from build123d import *

# Parameters (mm, degrees)
EXTRUDE_THIN1_DEPTH = 254
FILLET1_R           = 0.889


with BuildPart() as part:
    # Sketch1 → Extrude-Thin1 (new body)
    with BuildSketch(Plane.XY):
        with BuildLine():
            Line((0, 3.175), (0, 0))
            Line((0, 0), (-4.7625, 0))
            ThreePointArc((-4.7625, 0), (-6.154789008, 7.270660772), (-8.588987157, 14.261773425))
            ThreePointArc((-8.588987157, 14.261773425), (-11.515725494, 17.745797222), (-15.875, 19.05))
            Line((-15.875, 19.05), (-15.875, 25.4))
            Line((-15.875, 25.4), (0, 25.4))
            Line((0, 25.4), (0, 22.225))
            Line((0, 22.225), (-0.889, 22.225))
            Line((-0.889, 22.225), (-0.889, 24.511))
            Line((-0.889, 24.511), (-14.986, 24.511))
            Line((-14.986, 24.511), (-14.986, 19.894116096))
            ThreePointArc((-14.986, 19.894116096), (-10.661715447, 18.234912963), (-7.772953719, 14.614492048))
            ThreePointArc((-7.772953719, 14.614492048), (-5.400232677, 7.883084139), (-3.977402872, 0.889))
            Line((-3.977402872, 0.889), (-0.889, 0.889))
            Line((-0.889, 0.889), (-0.889, 3.175))
            Line((-0.889, 3.175), (0, 3.175))
        make_face()
    extrude(amount=-EXTRUDE_THIN1_DEPTH)

    # Fillet1
    fillet1_edges = [part.edges().sort_by_distance(p)[0] for p in [
        (0, 0, -127),
        (-4.7625, 0, -127),
        (-15.875, 19.05, -127),
        (-15.875, 25.4, -127),
        (0, 25.4, -127),
    ]]
    fillet(fillet1_edges, radius=FILLET1_R)


solid = part.part
For this review, take the finished solid that the model builds, in its own axes (mm). Give positions to 0.01 mm unless a question says otherwise; leave off trailing zeros. Loops run counter-clockwise (first coordinate to the right, second up) from the corner with the lowest first, then second, coordinate; pieces in that order, holes last. Notation, with made-up numbers: (-27.5, -38.5) -> (8.5, -38.5) arc R30 ccw to (8.5, -12.5) -> close; hole circle Ø8 at (43, 39). An arc over 180 degrees is marked (long way). One line per question, with ' | ' between items.
1) We need section C-C (y = 7.75). Write out the cut boundary in (x, z).
Resolved:
outline: (-6.29, -254) -> (-5.36, -254) -> (-5.36, 0) -> (-6.29, 0) -> close
2) To check wall thickness, follow probe 1 along Y at (x, z) = (-1, -93.5); probe 2 along X at (y, z) = (20, -115.5) (3 decimals); probe 3 along Y at (x, z) = (-8.25, -78.5). State the ranges of each line that lie inside material, in increasing order.
Resolved:
probe 1: y = 0 to 0.89, 24.51 to 25.4 | probe 2: x = -15.875 to -14.986 | probe 3: y = 13.46 to 15.56, 24.51 to 25.4
3) Insertion check: pin 1 Ø1 at (x, z) = (-0.5, -104.5) entering from -Y; pin 2 Ø4 at (y, z) = (12.5, -84) entering from +X; pin 3 Ø0.7 at (y, z) = (1.5, -123) entering from -X; pin 4 Ø5 at (x, z) = (-13.5, -71) entering from -Y. Each pin has a flat end and moves straight along its axis. Give the tip position at first contact, or say it passes through.
Resolved:
pin 1: stops at y = 0 | pin 2: stops at x = -6.2 | pin 3: stops at x = -5.01 | pin 4: stops at y = 17.38
4) We need section A-A (x = -11). Write out the cut boundary in (y, z).
Resolved:
outline: (17.38, -254) -> (18.47, -254) -> (18.47, 0) -> (17.38, 0) -> close; (24.51, -254) -> (25.4, -254) -> (25.4, 0) -> (24.51, 0) -> close
5) We need section B-B (z = -71). Write out the cut boundary in (x, y) (1 decimal), plus the area to 3 significant figures.
Resolved:
outline: (-15.9, 19.9) arc R0.9 ccw to (-15.1, 19) arc R7.9 cw to (-8.6, 14.3) arc R50.8 cw to (-4.9, 0.8) arc R0.9 ccw to (-4, 0) -> (-0.9, 0) arc R0.9 ccw to (0, 0.9) -> (0, 3.2) -> (-0.9, 3.2) -> (-0.9, 0.9) -> (-4, 0.9) arc R51.7 ccw to (-7.8, 14.6) arc R8.8 ccw to (-15, 19.9) -> (-15, 24.5) -> (-0.9, 24.5) -> (-0.9, 22.2) -> (0, 22.2) -> (0, 24.5) arc R0.9 ccw to (-0.9, 25.4) -> (-15, 25.4) arc R0.9 ccw to (-15.9, 24.5) -> close | area: 47.0 mm2
6) The part is to be moulded in two halves that separate along X. For faces 1 (the flat face through (-14.986, 22, -125)), 2 (the flat face through (-8, 24.511, -125)), 3 (the cylindrical face through (-11.139, 17.483, -125.222)), 4 (the cylindrical face through (-10.71, 18.27, -125.22)), say which applies: +X half, -X half, draft (parallel to the pull), parting line (faces both ways), or undercut.
Resolved:
face 1: undercut | face 2: undercut | face 3: -X half | face 4: +X half
